from build123d import *

# Parameters (mm, degrees)
SKETCH_1_W          = 194.6
SKETCH_1_H          = 17
EXTRUDE_1_DEPTH     = 3
FILLET_1_R          = 3
SKETCH_2_R          = 1.5
CUT_EXTRUDE_1_DEPTH = 3
SKETCH_3_R          = 1.5
CUT_EXTRUDE_2_DEPTH = 3
SKETCH_5_R          = 1.5
CUT_EXTRUDE_3_DEPTH = 3


with BuildPart() as part:
    # 草图1 → 凸台-拉伸1 (new body)
    with BuildSketch(Plane.XY):
        Rectangle(SKETCH_1_W, SKETCH_1_H)
    extrude(amount=EXTRUDE_1_DEPTH)

    # 圆角1
    fillet_1_edges = [part.edges().sort_by_distance(p)[0] for p in [
        (97.3, -8.5, 1.5),
        (-97.3, -8.5, 1.5),
        (-97.3, 8.5, 1.5),
        (97.3, 8.5, 1.5),
    ]]
    fillet(fillet_1_edges, radius=FILLET_1_R)

    # 草图2 → 切除-拉伸1 (cut)
    with BuildSketch(Plane.XY.offset(3)):
        with Locations((89.800213401, 5.5)):
            Circle(SKETCH_2_R)
        with Locations((89.800213401, -3.5)):
            Circle(SKETCH_2_R)
        with Locations((-89.8, -3.5)):
            Circle(SKETCH_2_R)
        with Locations((-89.8, 5.5)):
            Circle(SKETCH_2_R)
    extrude(amount=-CUT_EXTRUDE_1_DEPTH, mode=Mode.SUBTRACT)

    # 草图3 → 切除-拉伸2 (cut)
    with BuildSketch(Plane(origin=(0, 0, 0), x_dir=(-1, 0, 0), z_dir=(0, 0, -1))):
        with Locations((44.863842933, 5.5)):
            Circle(SKETCH_3_R)
        with Locations((34.863842933, 5.5)):
            Circle(SKETCH_3_R)
    extrude(amount=-CUT_EXTRUDE_2_DEPTH, mode=Mode.SUBTRACT)

    # 草图5 → 切除-拉伸3 (cut)
    with BuildSketch(Plane(origin=(0, 0, 0), x_dir=(-1, 0, 0), z_dir=(0, 0, -1))):
        with Locations((-45.188251481, 5.5)):
            Circle(SKETCH_5_R)
        with Locations((-35.188251481, 5.5)):
            Circle(SKETCH_5_R)
    extrude(amount=-CUT_EXTRUDE_3_DEPTH, mode=Mode.SUBTRACT)


solid = part.part
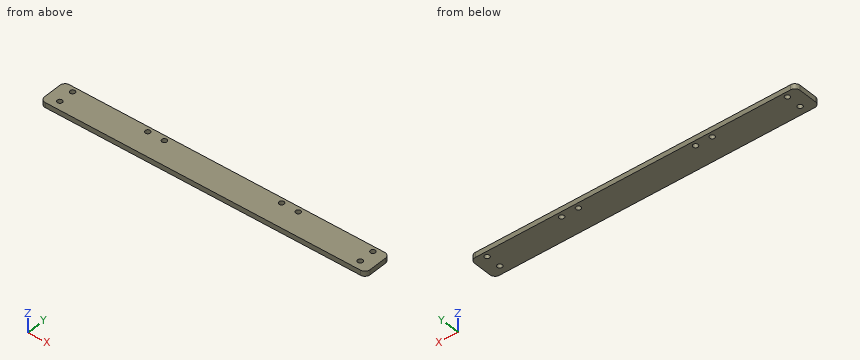
Work out the finished part from the listing and answer in its coordinate system (mm). Give positions to 0.01 mm unless a question says otherwise; leave off trailing zeros. Answer as CSV lines item,"result". Start each with the question number.
Q1. The part is cut by section A-A (z = 0.45). Give the number of separate pieces and of enclosed holes in the cut face, then the cut area to 3 significant figures.
Q2. Find the intervals of material crossed by L1, parallel to Y at x = -89.8, z = 1.6; L2, parallel to X at y = -2.5, z = 1.3, in increasing order. Write a range as [from, to].
Q3. Given pin 1 Ø2.5 at (x, y) = (-89.8, -3.5) entering from -Z, flat-ended and moving along its own axis, determine where the tip first touches the part or whether it passes through.
Check result:
1,separate pieces,"1"
1,enclosed holes,"8"
1,area,"3,240 mm²"
2,L1,"y = [-8.5, -5], [-2, 4], [7, 8.5]"
2,L2,"x = [-97.3, -90.92], [-88.68, 88.68], [90.92, 97.3]"
3,pin 1,"passes through"
